CAD build for the part. Positions are in the model's coordinates, mm. Face numbers are marked on the shaded views. Round coordinates to 2 decimals unless told otherwise and drop trailing zeros. Order: outer loops, then holes, each group sorted by start corner. A loop starts at its lowest first (then second) coordinate and runs counter-clockwise, first axis right, second up. Notation, with made-up numbers: M 26.5,12.5 L 57.5,12.5 A10 cw 57.5,29.5 Z; hole C -13,88.25 d3. An arc over 180 degrees is marked long. Answer as a JSON object with one key per item and string values.
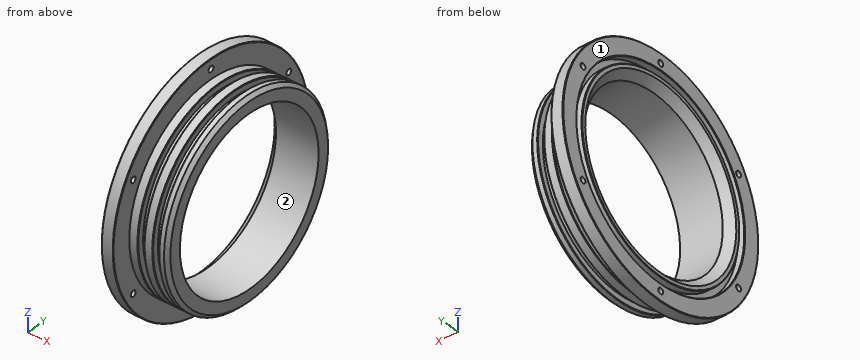
Autodesk Inventor part; units mm, degrees
ref_plane "YZ Plane" through (0, 0, 0) normal (1, 0, 0) x (0, 1, 0)
ref_plane "XZ Plane" through (0, 0, 0) normal (0, 1, 0) x (-1, 0, 0)
ref_plane "XY Plane" through (0, 0, 0) normal (0, 0, 1) x (1, 0, 0)
sketch "Sketch1" plane through (0, 0, 0) normal (0, 1, 0) x (-1, 0, 0)
  line L0 (0, 0) -> (4.445, 0)
  line L1 (0, 0) -> (0, -3.175)
  line L2 (0, -3.175) -> (-3.175, -3.175)
  line L3 (-3.175, -3.175) -> (-3.175, 0)
  line L4 (-3.175, 0) -> (-7.62, 0)
  line L5 (-7.62, 0) -> (-7.62, -3.175)
  line L6 (-7.62, -3.175) -> (-10.795, -3.175)
  line L7 (-10.795, -3.175) -> (-10.795, 0)
  line L8 (-10.795, 0) -> (-15.24, 0)
  line L9 (-15.24, 0) -> (-15.24, -7.62)
  line L10 (-15.24, -7.62) -> (4.445, -7.62)
  line L11 (4.445, -7.62) -> (4.445, 0)
  line L12 (-15.24, 0) -> (-15.24, -50.292) construction
  line L13 (-15.24, -50.292) -> (-2.54, -50.292) construction
  dimension "d0" = 4.445
  dimension "d1" = 3.175
  dimension "d2" = 3.175
  dimension "d3" = 4.445
  dimension "d4" = 3.175
  dimension "d5" = 4.445
  dimension "d6" = 7.62
  dimension "d7" = 50.292
  dimension "d38" = 12.7
revolve "Revolution1" add sketch "Sketch1" angle 360 about axis through (15.24, 0, -50.292) along (-1, 0, 0)
sketch "Sketch2" plane through (-4.445, 0, -50.292) normal (-1, 0, 0) x (0, 0, 1)
  circle A0 centre (0, 0) radius 60.198
  circle A1 centre (0, 0) radius 42.672
  dimension "d10" = 120.396
extrude "Extrusion1" add sketch "Sketch2" along normal blind 6.096
sketch "Sketch3" plane through (-10.541, 0, -50.292) normal (-1, 0, 0) x (0, 0, 1)
  circle A0 centre (0, 0) radius 48.5013
  circle A1 centre (0, 0) radius 51.6763
  circle A2 centre (0, 0) radius 42.672 construction
  dimension "d42" = 3.175
  dimension "d62" = 97.0026
extrude "Extrusion2" cut sketch "Sketch3" against normal blind 3.5306
chamfer "Chamfer1" distance 1.778 angle 45 1 edges at (15.24, 0, -100.584)
sketch "Sketch5" plane through (-10.541, 0, -50.292) normal (-1, 0, 0) x (0, 0, 1)
  circle A0 centre (0, 0) radius 55.245 construction
  circle A1 centre (0, 0) radius 42.672
  circle A2 centre (0, 0) radius 48.5013
  point P0 (-55.245, 0)
  point P1 (-27.6225, -47.8436)
  point P2 (27.6225, -47.8436)
  point P3 (55.245, 0)
  point P4 (27.6225, 47.8436)
  point P5 (-27.6225, 47.8436)
  dimension "d43" = 110.49
  dimension "d46" = 360
hole "Hole1" at (-10.541, 0, -105.537) at (-10.541, -47.8436, -77.9145) at (-10.541, -47.8436, -22.6695) at (-10.541, 0, 4.953) at (-10.541, 47.8436, -22.6695) at (-10.541, 47.8436, -77.9145) direction (1, 0, 0) diameter 3 end through all
chamfer "Chamfer2" distance 0.254 angle 45 8 edges at (0, 0, -100.584) (3.175, 0, -100.584) (7.62, 0, -100.584) (10.795, 0, -100.584) (-10.541, 0, -101.9683) (-10.541, 0, -98.7933) (-10.541, 0, -110.49) (-4.445, 0, -110.49)
sketch "Sketch8" plane through (-10.541, 0, -50.292) normal (-1, 0, 0) x (0, 0, 1)
  circle A0 centre (0, 0) radius 48.2473
  point P0 (50.292, 0)
chamfer "Chamfer3" distance 3.81 angle 45 1 edges at (-10.541, 0, -92.964)
properties part number "Oring Fitting Dome V2"
Item 1: Saw through at B-B on y = 0. State how many separate pieces and enclosed holes the cut face has, and give its area (3 significant figures).
Worked answers:
{"separate pieces": "4", "enclosed holes": "0", "area": "396 mm2"}
Item 2: Saw through at A-A on x = 1.5. List the corners of the cut face in (y, z) (3 decimals), and give its area (3 significant figures).
Worked answers:
{"outline": "C 0,-50.292 d94.234; hole C 0,-50.292 d85.344", "area": "1,250 mm2"}
Item 3: Drop flat-ended pins along their axis: pin 1 Ø6 at (x, z) = (11, -35.5) entering from -Y; pin 2 Ø5 at (y, z) = (-47.84, -22.67) entering from +X (3 decimals); pin 3 Ø2.5 at (y, z) = (-47.84, -77.91) entering from +X; pin 4 Ø8 at (y, z) = (44.5, -78.5) entering from +X. Give the stop position or say it passes through.
Worked answers:
{"pin 1": "stops at y = -48.89", "pin 2": "stops at x = -4.445", "pin 3": "passes through", "pin 4": "stops at x = 15.07"}
Item 4: Two-plate mould, pull along Y, no slides. Class the marked faces 1 and 2: released by +Y, released by -Y, zero draft, split by the parting line, or undercut.
Worked answers:
{"face 1": "zero draft", "face 2": "undercut"}
Item 5: Wall check: line 1 along Y through (x, z) = (-6.75, -49); line 2 along X through (y, z) = (34.5, -13) (3 decimals); line 3 along Z through (x, y) = (12, -1). Give the ranges that are in metal, low to high. Write a range as [from, to].
Worked answers:
{"line 1": "y = [-60.18, -42.67], [42.67, 60.18]", "line 2": "x = [-7.01, -4.445]", "line 3": "z = [-100.57, -92.95], [-7.63, -0.01]"}
